from build123d import *

# Parameters (mm, degrees)
ESQUISSE1_W                  = 40
ESQUISSE1_H                  = 18
BOSS_EXTRU_1_DEPTH           = 12
ESQUISSE2_W                  = 40
ESQUISSE2_H                  = 12
BOSS_EXTRU_2_DEPTH           = 10
ENL_V_MAT_EXTRU_1_DEPTH      = 12
ESQUISSE4_R                  = 2.5
ENL_V_MAT_EXTRU_2_DEPTH      = 28
ESQUISSE5_R                  = 2.5
ENL_V_MAT_EXTRU_3_DEPTH      = 12
ESQUISSE6_R                  = 4
ENL_V_MAT_EXTRU_5_DEPTH      = 12
ESQUISSE7_W                  = 12
ESQUISSE7_H                  = 18
BOSS_EXTRU_3_DEPTH           = 15
ESQUISSE8_W                  = 12
ESQUISSE8_H                  = 18
BOSS_EXTRU_4_DEPTH           = 15
ESQUISSE9_R                  = 2.5
ENL_V_MAT_EXTRU_6_DEPTH      = 12
CONG_1_R                     = 2
ENL_V_MAT_EXTRU_7_DEPTH      = 10
ENL_V_MAT_EXTRU_7_DEPTH_BACK = 27
ESQUISSE11_W                 = 15
ESQUISSE11_H                 = 16.6984892
CONG_2_R                     = 2


# Some blends are built 0.0001 mm under size
with BuildPart() as part:
    # Esquisse1 → Boss.-Extru.1 (new body)
    with BuildSketch(Plane.XY):
        with Locations((3.185612757, 0.725848564)):
            Rectangle(ESQUISSE1_W, ESQUISSE1_H)
    extrude(amount=BOSS_EXTRU_1_DEPTH)

    # Esquisse2 → Boss.-Extru.2 (add)
    with BuildSketch(Plane.XZ.offset(8.274151436)):
        with Locations((3.185612757, 6)):
            Rectangle(ESQUISSE2_W, ESQUISSE2_H)
    extrude(amount=BOSS_EXTRU_2_DEPTH)

    # Esquisse3 → Enlèv. mat.-Extru.1 (cut)
    with BuildSketch(Plane.XY.offset(12)):
        with BuildLine():
            Line((-2.864387243, -18.274151436), (9.235612757, -18.274151436))
            ThreePointArc((9.235612757, -18.274151436), (3.185612757, -12.224151436), (-2.864387243, -18.274151436))
        make_face()
    extrude(amount=-ENL_V_MAT_EXTRU_1_DEPTH, mode=Mode.SUBTRACT)

    # Esquisse4 → Enlèv. mat.-Extru.2 (cut)
    with BuildSketch(Plane.XZ.offset(18.274151436)):
        with Locations(Location((-9.839387243, 6, 0), (0, 0, 270))):
            Circle(ESQUISSE4_R)
        with Locations(Location((16.210612757, 6, 0), (0, 0, 270))):
            Circle(ESQUISSE4_R)
    extrude(amount=-ENL_V_MAT_EXTRU_2_DEPTH, mode=Mode.SUBTRACT)

    # Esquisse5 → Enlèv. mat.-Extru.3 (cut)
    with BuildSketch(Plane.XY.offset(12)):
        with Locations((3.185612757, 0.725848564)):
            Circle(ESQUISSE5_R)
    extrude(amount=-ENL_V_MAT_EXTRU_3_DEPTH, mode=Mode.SUBTRACT)

    # Esquisse6 → Enlèv. mat.-Extru.5 (cut)
    with BuildSketch(Plane(origin=(0, 9.725848564, 0), x_dir=(1, 0, 0), z_dir=(0, 1, 0))):
        with Locations(Location((16.210612757, -6, 0), (0, 0, 270))):
            Circle(ESQUISSE6_R)
        with Locations(Location((-9.839387243, -6, 0), (0, 0, 270))):
            Circle(ESQUISSE6_R)
    extrude(amount=-ENL_V_MAT_EXTRU_5_DEPTH, mode=Mode.SUBTRACT)

    # Esquisse7 → Boss.-Extru.3 (add)
    with BuildSketch(Plane.ZY.offset(16.814387243)):
        with Locations((6, 0.725848564)):
            Rectangle(ESQUISSE7_W, ESQUISSE7_H)
    extrude(amount=BOSS_EXTRU_3_DEPTH)

    # Esquisse8 → Boss.-Extru.4 (add)
    with BuildSketch(Plane(origin=(23.185612757, 0, 0), x_dir=(0, 0, -1), z_dir=(1, 0, 0))):
        with Locations((-6, 0.725848564)):
            Rectangle(ESQUISSE8_W, ESQUISSE8_H)
    extrude(amount=BOSS_EXTRU_4_DEPTH)

    # Esquisse9 → Enlèv. mat.-Extru.6 (cut)
    with BuildSketch(Plane.XY.offset(12)):
        with Locations((-24.314387243, 0.725848564)):
            Circle(ESQUISSE9_R)
        with Locations((30.685612757, 0.725848564)):
            Circle(ESQUISSE9_R)
    extrude(amount=-ENL_V_MAT_EXTRU_6_DEPTH, mode=Mode.SUBTRACT)

    # Congé1
    cong_1_edges = [part.edges().sort_by_distance(p)[0] for p in [
        (3.185612757, 9.725848564, 0),
        (23.185612757, -13.274151436, 0),
        (-16.814387243, -13.274151436, 0),
        (-16.814387243, -8.274151436, 6),
        (-24.314387243, -8.274151436, 0),
        (-31.814387243, 0.725848564, 0),
        (-31.814387243, -8.274151436, 6),
        (-31.814387243, 9.725848564, 6),
        (30.685612757, -8.274151436, 0),
        (23.185612757, -8.274151436, 6),
        (38.185612757, 0.725848564, 0),
        (38.185612757, 9.725848564, 6),
        (38.185612757, -8.274151436, 6),
    ]]
    fillet(cong_1_edges, radius=CONG_1_R - 0.0001)  # a hair under: the kernel refuses the full size

    # Esquisse11 → Enlèv. mat.-Extru.7 (cut, two sides: drawn at the far end of the back side and taken through both)
    with BuildSketch(Plane.XZ.offset(8.274151436).offset(-ENL_V_MAT_EXTRU_7_DEPTH_BACK)):
        with Locations((30.685612757, 5.475380595)):
            Rectangle(ESQUISSE11_W, ESQUISSE11_H)
    extrude(amount=ENL_V_MAT_EXTRU_7_DEPTH + ENL_V_MAT_EXTRU_7_DEPTH_BACK, mode=Mode.SUBTRACT)

    # Congé2
    # the kernel refuses this fillet: 2 mm, written as the material it takes off along each edge
    with BuildSketch(Plane(origin=(23.185612757, 9.725848564, 1.9999), x_dir=(-0.999999998749875, 5.00025000614922e-05, 0), z_dir=(0, 0, 1))) as cong_2_piece_1:
        with BuildLine():
            CenterArc((1.999799997, 1.999999997), CONG_2_R, 180.002864932, 90)
            Line((-0.0002, 1.999899992), (-0.0402, 1.999897992))
            ThreePointArc((-0.0402, 1.999897992), (-0.04005, 0.999947999), (-0.04, -2e-06))
            Line((-0.04, -2e-06), (2e-06, -0.04))
            ThreePointArc((2e-06, -0.04), (0.999951999, -0.03995), (1.999902003, -0.04))
            Line((1.999902003, -0.04), (1.999900003, 0))
        make_face()
    extrude(amount=14.999850006, mode=Mode.SUBTRACT)
    with BuildSketch(Plane(origin=(23.185612757, 7.725948564, 1.9999), x_dir=(0, 1, 0), z_dir=(0, 0, 1))) as cong_2_piece_2:
        with BuildLine():
            CenterArc((0, 1.9999), CONG_2_R, 270, 90)
            Line((2, 1.9999), (2.04, 1.9999))
            ThreePointArc((2.04, 1.9999), (2.0399, 0.99995), (2.0399, 0))
            Line((2.0399, 0), (1.9999, -0.04))
            ThreePointArc((1.9999, -0.04), (0.99995, -0.04), (0, -0.0401))
            Line((0, -0.0401), (0, -0.0001))
        make_face()
    revolve(axis=Axis((23.185612757, 7.725948564, 1.9999), (-1, 0, 0)), revolution_arc=90, mode=Mode.SUBTRACT)
    with BuildSketch(Plane(origin=(23.185612757, -11.809873032, 0), x_dir=(-0.999999998749875, 0, -5.000250006249136e-05), z_dir=(0, 1, 0))) as cong_2_piece_3:
        with BuildLine():
            CenterArc((1.999799998, 1.999999997), CONG_2_R, 180.002864932, 90)
            Line((-0.0002, 1.999899992), (-0.0402, 1.999897992))
            ThreePointArc((-0.0402, 1.999897992), (-0.04005, 0.999947999), (-0.04, -2e-06))
            Line((-0.04, -2e-06), (2e-06, -0.04))
            ThreePointArc((2e-06, -0.04), (0.999951999, -0.03995), (1.999902003, -0.04))
            Line((1.999902003, -0.04), (1.999900003, 0))
        make_face()
    extrude(amount=19.535821596, mode=Mode.SUBTRACT)


solid = part.part
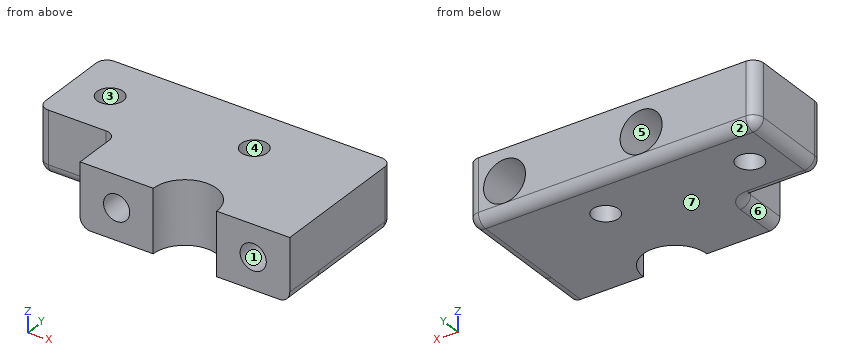
Design review of the part built by this model. Coordinates are the model's own, in mm. Face numbers are marked on the shaded views. A direction names the side the tool comes from. Coordinates: 2 decimals unless noted, no trailing zeros. Loops run counter-clockwise (first coordinate to the right, second up) from the corner with the lowest first, then second, coordinate; pieces in that order, holes last. Notation, with made-up numbers: M 49.25,57 L 60.25,57 A12 ccw 60.25,74 Z; hole C 66,-10.75 d10. An arc over 180 degrees is marked long. Use one line per item in the form item = value.
(1) Consider section C-C (z = 6). Give the number of separate pieces and of enclosed holes in the cut face, and give its area (3 significant figures).
Return value:
separate_pieces = 3
enclosed_holes = 2
area = 940 mm2
(2) Clearance check with flat-ended pins moving along their axes: P1, Ø6.5, axis at x = -9.84, z = 6, coming from the +Y side; P2, Ø2.5, axis at y = -13.5, z = 9, coming from the -X side; P3, Ø6.5, axis at x = 17, z = 5, coming from the +Y side. State where each tip first meets the part, or that it passes through.
Return value:
P1 = -2.27
P2 = -16.81
P3 = 9.73
(3) For line 1 along X through (y, z) = (6.5, 6); line 2 along X through (y, z) = (-9.75, 6); line 3 along X through (y, z) = (0, 6), list the stretches that pass through material, from the lowest coordinate up. Write a range as from..to.
Return value:
line_1 = -31.81..-13.84, -5.84..12.21, 20.21..23.19
line_2 = -16.88..-12.34, -7.34..13.71, 18.71..23.19
line_3 = -31.81..-26.71, -21.92..-13.84, -5.84..0.79, 5.58..12.21, 20.21..23.19
(4) Consider section B-B (x = -8). Write out the cut boundary in (y, z), and give its area (3 significant figures).
Return value:
outline = M -18.27,0 L 7.73,0 A2 ccw 9.73,2 L 9.73,2.45 L -2.27,2.45 L -2.27,4.31 L -18.27,4.31 Z; M -18.27,7.69 L -2.27,7.69 L -2.27,9.55 L 9.73,9.55 L 9.73,12 L -18.27,12 Z
area = 196 mm2
(5) Consider section D-D (y = 6.75). Write out the cut boundary in (x, z), and give its area (3 significant figures).
Return value:
outline = M -31.81,2 A2 ccw -29.81,0 L 21.21,0 A2 ccw 23.19,1.98 L 23.19,12 L -31.81,12 Z; hole C -9.84,6 d8; hole C 16.21,6 d8
area = 558 mm2
(6) Consider section A-A (y = -14.75). Write out the cut boundary in (x, z), and give its area (3 significant figures).
Return value:
outline = M -16.81,2 A2 ccw -14.81,0 L -1.73,0 L -1.73,12 L -16.81,12 Z; M 8.1,0 L 21.19,0 A2 ccw 23.19,2 L 23.19,12 L 8.1,12 Z; hole C -9.84,6 d5; hole C 16.21,6 d5
area = 321 mm2
(7) For the marked faces 5, 6 and 7, list the 3-axis set-ups (+Z, -Z, +X, -X, +Y, -Y) from which the entire face can be reached by the end or side of a thin tool; tool diameter is ignored.
Return value:
face_5 = +Y
face_6 = -Z, -X, -Y
face_7 = -Z, +X, -X, +Y, -Y
(8) Draft analysis for pull direction Y (two halves, no side actions). For the marked faces 1, 2, 3 and 4, state which applies: pulls with the +Y half, pulls with the -Y half, needs draft (parallel to the pull), parting line crosses it, or undercut.
Return value:
face_1 = needs draft
face_2 = pulls with the +Y half
face_3 = undercut
face_4 = undercut
